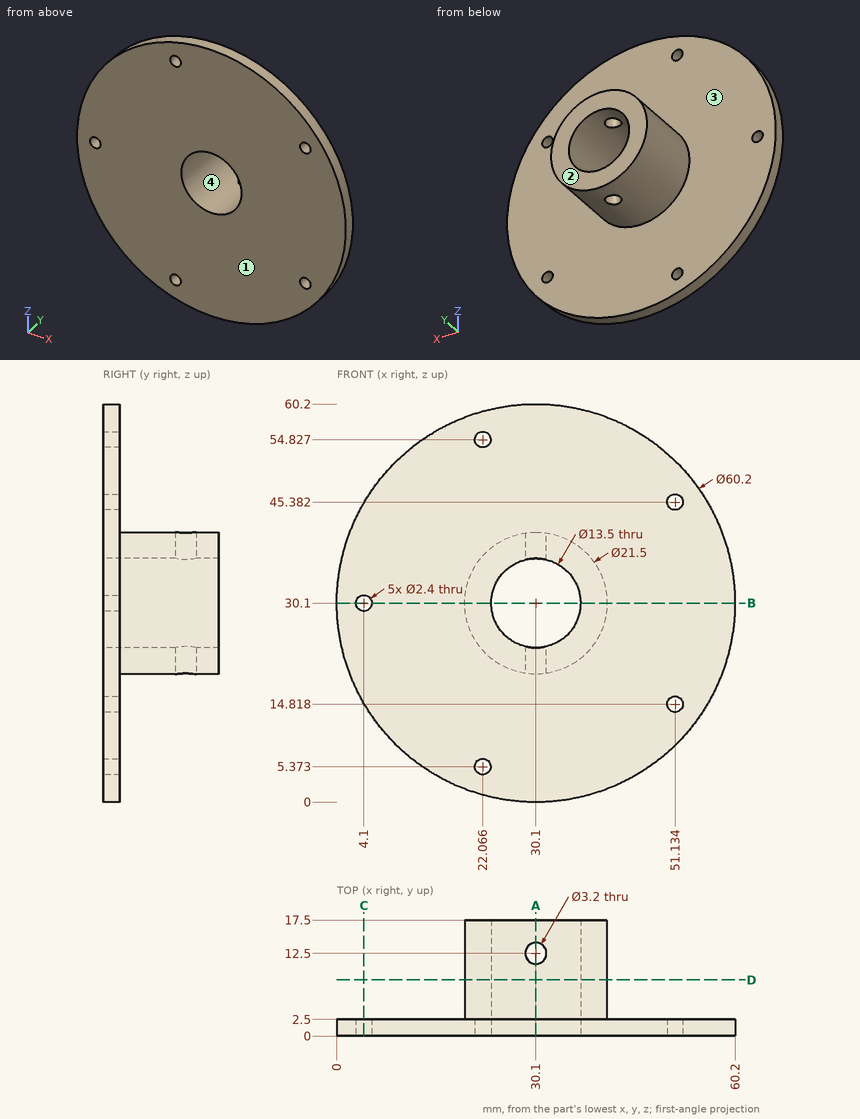
Geometry: see drawing. Coordinates: mm, zero at the bounding-box minimum. A direction names the side the tool comes from. Coordinates: 2 decimals unless noted, no trailing zeros. Loops run counter-clockwise (first coordinate to the right, second up) from the corner with the lowest first, then second, coordinate; pieces in that order, holes last. Notation, with made-up numbers: M -22.75,-22 L 16.25,-22 A26 ccw 16.25,16 Z; hole C 61,42.25 d8. An arc over 180 degrees is marked long. Answer in a Markdown table with one row per item.
1. Section C-C, the plane x = 4.1. Output: boundary loops of the cut face in (y, z).
Response:
| item | result |
|---|---|
| outline | M 0,14.93 L 2.5,14.93 L 2.5,28.9 L 0,28.9 Z; M 0,31.3 L 2.5,31.3 L 2.5,45.27 L 0,45.27 Z |
2. Section B-B, the plane z = 30.1. Output: boundary loops of the cut face in (x, y).
Response:
| item | result |
|---|---|
| outline | M 0,0 L 2.9,0 L 2.9,2.5 L 0,2.5 Z; M 5.3,0 L 23.35,0 L 23.35,17.5 L 19.35,17.5 L 19.35,2.5 L 5.3,2.5 Z; M 36.85,0 L 60.2,0 L 60.2,2.5 L 40.85,2.5 L 40.85,17.5 L 36.85,17.5 Z |
3. Reachability of the marked faces 3 and 4 from +Z, -Z, +X, -X, +Y, -Y: full face, straight path, thin tool, end or side. Return the list, or none.
Response:
| item | result |
|---|---|
| face 3 | +Y |
| face 4 | +Y, -Y |
4. First-contact query: pin 1 (6 mm diameter, centred on y = 8.5, z = 23.5, fed in from +X); pin 2 (3 mm diameter, centred on x = 22.07, z = 54.83, fed in from +Y); pin 3 (4 mm diameter, centred on x = 14, y = 2, fed in from -Z). Flat tips, straight axial feed; report the tip coordinate or a pass-through.
Response:
| item | result |
|---|---|
| pin 1 | stops at x = 40.23 |
| pin 2 | stops at y = 2.5 |
| pin 3 | stops at z = 3.51 |
5. Section D-D, the plane y = 8.5. Output: boundary loops of the cut face in (x, z), then the cut area to 3 significant figures.
Response:
| item | result |
|---|---|
| outline | C 30.1,30.1 d21.5; hole C 30.1,30.1 d13.5 |
| area | 220 mm2 |
6. Material intervals for line 1 (X direction, y = 1.4, z = 30.1); line 2 (Y direction, x = 30, z = 22); line 3 (Y direction, x = 40.5, z = 43), sorted ascending.
Response:
| item | result |
|---|---|
| line 1 | x = 0 to 2.9, 5.3 to 23.35, 36.85 to 60.2 |
| line 2 | y = 0 to 10.9, 14.1 to 17.5 |
| line 3 | y = 0 to 2.5 |
7. Draft query along Y for the marked faces 1 and 2. Return one class per face: pulls with the +Y half, pulls with the -Y half, needs draft (parallel to the pull), parting line crosses it, or undercut.
Response:
| item | result |
|---|---|
| face 1 | pulls with the -Y half |
| face 2 | pulls with the +Y half |
8. Section A-A, the plane x = 30.1. Output: boundary loops of the cut face in (y, z), then the cut area to 3 significant figures.
Response:
| item | result |
|---|---|
| outline | M 0,0 L 2.5,0 L 2.5,19.35 L 10.9,19.35 L 10.9,23.35 L 0,23.35 Z; M 0,36.85 L 10.9,36.85 L 10.9,40.85 L 2.5,40.85 L 2.5,60.2 L 0,60.2 Z; M 14.1,19.35 L 17.5,19.35 L 17.5,23.35 L 14.1,23.35 Z; M 14.1,36.85 L 17.5,36.85 L 17.5,40.85 L 14.1,40.85 Z |
| area | 211 mm2 |
